```python
from build123d import *

# Parameters (mm, degrees)
F0_R     = 25.4
F0_R_2   = 10.795
F1_DEPTH = 177.8
F2_R     = 25.4
F3_DEPTH = 50.8
F4_SIZE2 = 25.4
F4_SIZE  = 50.8


with BuildPart() as f1:
    # F0 (on Top) → F1 (new body)
    with BuildSketch(Plane.XY):
        with Locations((0, -4.202133)):
            Circle(F0_R)
        with Locations((0, -4.202133)):
            Circle(F0_R_2, mode=Mode.SUBTRACT)
    extrude(amount=F1_DEPTH)

    # F2 (on face) → F3 (join)
    with BuildSketch(Plane.XY.offset(177.8)):
        with Locations((0, -4.202133)):
            Circle(F2_R)
    extrude(amount=F3_DEPTH)

    # F4
    f4_edges = [f1.edges().sort_by_distance(p)[0] for p in [
        (-25.4, -4.202133, 228.6),
    ]]
    chamfer(f4_edges, length=F4_SIZE, length2=F4_SIZE2)


solid = f1.part
```
Could you check a few things on this model? Use its own coordinates, in mm. A direction names the side the tool comes from. Give positions to 0.01 mm unless a question says otherwise; leave off trailing zeros. Loops run counter-clockwise (first coordinate to the right, second up) from the corner with the lowest first, then second, coordinate; pieces in that order, holes last. Notation, with made-up numbers: (26.25, 7.25) - (56.25, 7.25) arc R30 ccw to (56.25, 35.25) - close; hole circle Ø1 at (48, 10.5). An arc over 180 degrees is marked (long way). Use one line per item in the form item = value.
1. I'm going to push flat-ended pins straight in: pin 1 Ø5 at (x, y) = (5.5, 14) entering from -Z; pin 2 Ø1 at (x, z) = (8, 129.5) entering from +Y; pin 3 Ø6 at (x, z) = (12.5, 173) entering from +Y; pin 4 Ø10 at (x, y) = (9.5, -19.5) entering from +Z. Where does each tip first touch, or does it pass through?
Response values:
pin_1 = 0
pin_2 = 20.07
pin_3 = 19.35
pin_4 = 202.58
2. I want a section at A-A (z = 118.5). Please give me the cut outline in (x, y) (3 decimals).
Response values:
outline = circle Ø50.8 at (0, -4.202); hole circle Ø21.59 at (0, -4.202)
3. I want a section at B-B (z = 212.5). Please give me the cut outline in (x, y), and give its area (3 significant figures).
Response values:
outline = circle Ø16.1 at (0, -4.2)
area = 204 mm²
4. Thinking about a two-plate mould opening in X: for faces 3 (the face through (-7.7, -10.1, 209.2)), 4 (the face through (11, -4, 0)), 5 (the face through (-8.567, -10.771, 87.655)), which applies, released by +X, released by -X, zero draft, split by the parting line, or undercut?
Response values:
face_3 = split by the parting line
face_4 = zero draft
face_5 = undercut
5. On a 3-axis mill with a long thin cutter (end or side, diameter ignored), from which of +Z, -Z, +X, -X, +Y, -Y can I reach the whole of each face in a straight line? I mean faces 1 (the face through (-3.31, 20.98, 87.66)), 2 (the face through (0, -4, 177.8)). Say none if no direction works.
Response values:
face_1 = +Z, -Z
face_2 = -Z
6. I need wall thicknesses on probe 1 along X at (y, z) = (-3.5, 165); probe 2 along Y at (x, z) = (0, 41); probe 3 along Y at (x, z) = (-1, 75). Which ranges of each line are inside material? Lowest first, please.
Response values:
probe_1 = -25.39 to -10.77, 10.77 to 25.39
probe_2 = -29.6 to -15, 6.59 to 21.2
probe_3 = -29.58 to -14.95, 6.55 to 21.18
